Can you work these out from the model? Positions are in its coordinate system, mm. Face numbers are marked on the shaded views. A direction names the side the tool comes from. Give positions to 0.01 mm unless a question says otherwise; leave off trailing zeros. Write each loop counter-clockwise with the first axis right and the second up, starting at its lowest first coordinate (ties: lowest second). Pieces come first, ordered by that corner, then holes.
1. Suppose I cut it at A-A (y = 1.25). Please give me the cut outline in (x, z), and give its area (3 significant figures).
2. Suppose I cut it at B-B (z = 1.45). Please give me the cut outline in (x, y), and give its area (3 significant figures).
3. Thinking about a two-plate mould opening in Y: for the marked faces 1, 2 and 3, which applies, pulls with the +Y half, pulls with the -Y half, needs draft (parallel to the pull), parting line crosses it, or undercut?
4. I'm going to push flat-ended pins straight in: pin 1 (1.6 mm diameter, centred on x = 4.5, z = 3.5, fed in from +Y); pin 2 (1.5 mm diameter, centred on x = -2, y = 0.5, fed in from +Z); pin 3 (1.5 mm diameter, centred on x = -0.5, z = 1.5, fed in from +Y); pin 4 (2 mm diameter, centred on x = -3, y = 0.5, fed in from +Z). Where does each tip first touch, or does it pass through?
5. Suppose I cut it at D-D (y = -1.5). Please give me the cut outline in (x, z).
6. Suppose I cut it at C-C (x = -2). Please give me the cut outline in (y, z).
7. On a 3-axis mill with a long thin cutter (end or side, diameter ignored), from which of +Z, -Z, +X, -X, +Y, -Y can I reach the whole of each face in a straight line? I mean the marked faces 4, 5 and 6. Say none if no direction works.
8. If I drill on probe 1 along Y at (x, z) = (4.4, 4); probe 2 along X at (y, z) = (0.25, 3); probe 3 along Z at (x, y) = (-0.25, 0.75), over which ranges is the centre line in solid material (lowest first)?
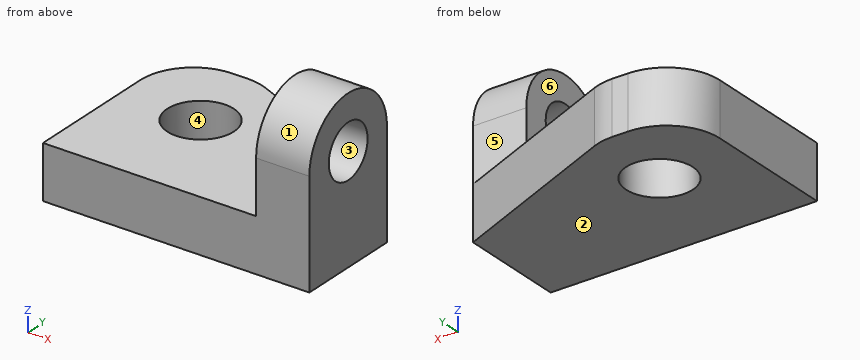
Autodesk Inventor part; units mm, degrees
ref_plane "YZ Plane" through (0, 0, 0) normal (1, 0, 0) x (0, 1, 0)
ref_plane "XZ Plane" through (0, 0, 0) normal (0, 1, 0) x (-1, 0, 0)
ref_plane "XY Plane" through (0, 0, 0) normal (0, 0, 1) x (1, 0, 0)
sketch "Boceto1" plane through (0, 0, 0) normal (0, 0, 1) x (1, 0, 0)
  line L0 (-5, -3.5) -> (5, -3.5)
  line L1 (5, -3.5) -> (5, 0.5)
  line L2 (-2.4105, 3.5) -> (-3, 3.5)
  line L3 (-5, 1.5) -> (-5, -3.5)
  line L4 (-5, -3.5) -> (5, 3.5) construction
  line L5 (5, -3.5) -> (-5, 3.5) construction
  arc A0 (-3, 3.5) -> (-5, 1.5) centre (-3, 1.5) ccw
  line L6 (-1.6227, 3.3383) -> (5, 0.5)
  circle A1 centre (-2, 0.5) radius 1.25
  arc A2 (-1.6227, 3.3383) -> (-2.4105, 3.5) centre (-2.4105, 1.5) ccw
  point P0 (0, 0)
  point P1 (-2, 3.5)
  dimension "d0" = 10
  dimension "d1" = 7
  dimension "d2" = 2
  dimension "d3" = 7
  dimension "d4" = 3
  dimension "d5" = 2.5
  dimension "d6" = 3
  dimension "d7" = 4
  dimension "d10" = 2
extrude "Extrusión1" add sketch "Boceto1" along normal blind 2
sketch "Boceto2" plane through (5, -3.5, 0) normal (1, 0, 0) x (0, 0, -1)
  line L0 (0, 0) -> (-2, 0)
  line L1 (0, 0) -> (-4, 0)
  line L2 (-6, 2) -> (-6, 2)
  line L3 (-4, 4) -> (0, 4)
  line L4 (0, 4) -> (0, 0)
  circle A0 centre (-4, 2) radius 1
  arc A1 (-4, 4) -> (-6, 2) centre (-4, 2) ccw
  arc A2 (-6, 2) -> (-4, 0) centre (-4, 2) ccw
  point P0 (0, 3.5)
  point P1 (-6, 4)
  point P2 (-6, 0)
  dimension "d11" = 6
  dimension "d12" = 4
  dimension "d13" = 2
  dimension "d14" = 2
  dimension "d15" = 2
  dimension "d16" = 2
extrude "Extrusión2" add sketch "Boceto2" against normal blind 2
sketch "Boceto3" plane through (3, -3.5, 0) normal (-1, 0, 0) x (0, 0, -1)
  point P0 (0, 3.5)
properties part number "Lab2A01209499P15"
Checks:
1. outline: (-5, 0) - (-3, 0) - (-3, 2) - (-5, 2) - close; (-1, 0) - (3.25, 0) - (3.25, 2) - (-1, 2) - close
1. area: 12.5 mm2
2. outline: (-5, -3.5) - (5, -3.5) - (5, 0.5) - (-1.62, 3.34) arc R2 ccw to (-2.41, 3.5) - (-3, 3.5) arc R2 ccw to (-5, 1.5) - close; hole circle Ø2.5 at (-2, 0.5)
2. area: 53.7 mm2
3. face 1: parting line crosses it
3. face 2: needs draft
3. face 3: undercut
4. pin 1: stops at y = 0.5
4. pin 2: passes through
4. pin 3: stops at y = 3.18
4. pin 4: stops at z = 2
5. outline: (-5, 0) - (5, 0) - (5, 3) - (3, 3) - (3, 2) - (-5, 2) - close; (3, 5) - (5, 5) - (5, 6) - (3, 6) - close
6. outline: (-3.5, 0) - (-0.75, 0) - (-0.75, 2) - (-3.5, 2) - close; (1.75, 0) - (3.46, 0) - (3.46, 2) - (1.75, 2) - close
7. face 4: +Z, -Z
7. face 5: +Z, +X, -X, +Y
7. face 6: +Z, -X, +Y, -Y
8. probe 1: y = -3.5 to -2.5, -0.5 to 0.5
8. probe 2: x = 3 to 5
8. probe 3: z = 0 to 2
